For this review, take the finished solid that the model builds, in its own axes (mm). A direction names the side the tool comes from. Give positions to 0.01 mm unless a question says otherwise; leave off trailing zeros. Order: outer loops, then holes, each group sorted by start corner. A loop starts at its lowest first (then second) coordinate and runs counter-clockwise, first axis right, second up. Notation, with made-up numbers: (71, 40.25) -> (87, 40.25) arc R14 cw to (87, 66.25) -> close; hole circle Ø3 at (88.25, 51). An arc over 180 degrees is marked (long way). Return JSON: item names as keys, results as strings. Group by question number.
1) Insertion check: P1, Ø4, axis at x = 28, y = -2.5, coming from the +Z side; P2, Ø1, axis at x = 16, z = -2, coming from the +Y side; P3, Ø1, axis at x = 9, y = 2.5, coming from the -Z side. Each pin has a flat end and moves straight along its axis. Give the tip position at first contact, or say it passes through.
2) For faces 1 (the face through (23.69, -2.64, -2.87)), 2 (the face through (13.119, -3.545, -0.465)), list the 3-axis set-ups (+Z, -Z, +X, -X, +Y, -Y) from which the entire face can be reached by the end or side of a thin tool; tool diameter is ignored.
3) Add section A-A (x = 15). Give the boundary of the cut face in (y, z) (3 decimals), then the cut area to 3 significant figures.
4) To check wall thickness, follow line 1 along Z through (x, y) = (2, -1.75); line 2 along Z through (x, y) = (5, -1); line 3 along Y through (x, z) = (2.5, 0.5). State the ranges of each line that lie inside material, in increasing order.
from build123d import *


with BuildPart() as part:
    # Esboço1 → Revolução1 (revolve)
    with BuildSketch(Plane.XY, mode=Mode.PRIVATE) as revolu_o1_sk:
        with BuildLine():
            Line((0, 0), (0, 1.75))
            Line((0, 1.75), (5.014146291, 3.575))
            Line((5.014146291, 3.575), (21, 3.575))
            Line((21, 3.575), (21, 3.9))
            Line((21, 3.9), (26.3, 3.9))
            ThreePointArc((26.3, 3.9), (30.103104016, 3.114541229), (33.456230179, 1.155691933))
            ThreePointArc((33.456230179, 1.155691933), (33.857266604, 0.638613628), (34, 0))
            Line((34, 0), (0, 0))
        make_face()
    revolve(revolu_o1_sk.sketch.rotate(Axis((0, 0, 0), (1, 0, 0)), 90), axis=Axis((0, 0, 0), (1, 0, 0)))


solid = part.part
Evaluation:
{
 "1": {"P1": "z = 3.77", "P2": "y = 3.25", "P3": "z = -2.96"},
 "2": {"face 1": "+X, -X", "face 2": "-X"},
 "3": {"outline": "circle Ø7.15 at (0, 0)", "area": "40.2 mm^2"},
 "4": {"line 1": "-1.75 to 1.75", "line 2": "-3.43 to 3.43", "line 3": "-2.61 to 2.61"}
}
